Source: three-view drawing plus pictorial views. Frame: mm from the lowest corner of the part. A direction names the side the tool comes from. Give positions to 0.01 mm unless a question says otherwise; leave off trailing zeros. Order: outer loops, then holes, each group sorted by start corner. A loop starts at its lowest first (then second) coordinate and runs counter-clockwise, first axis right, second up.
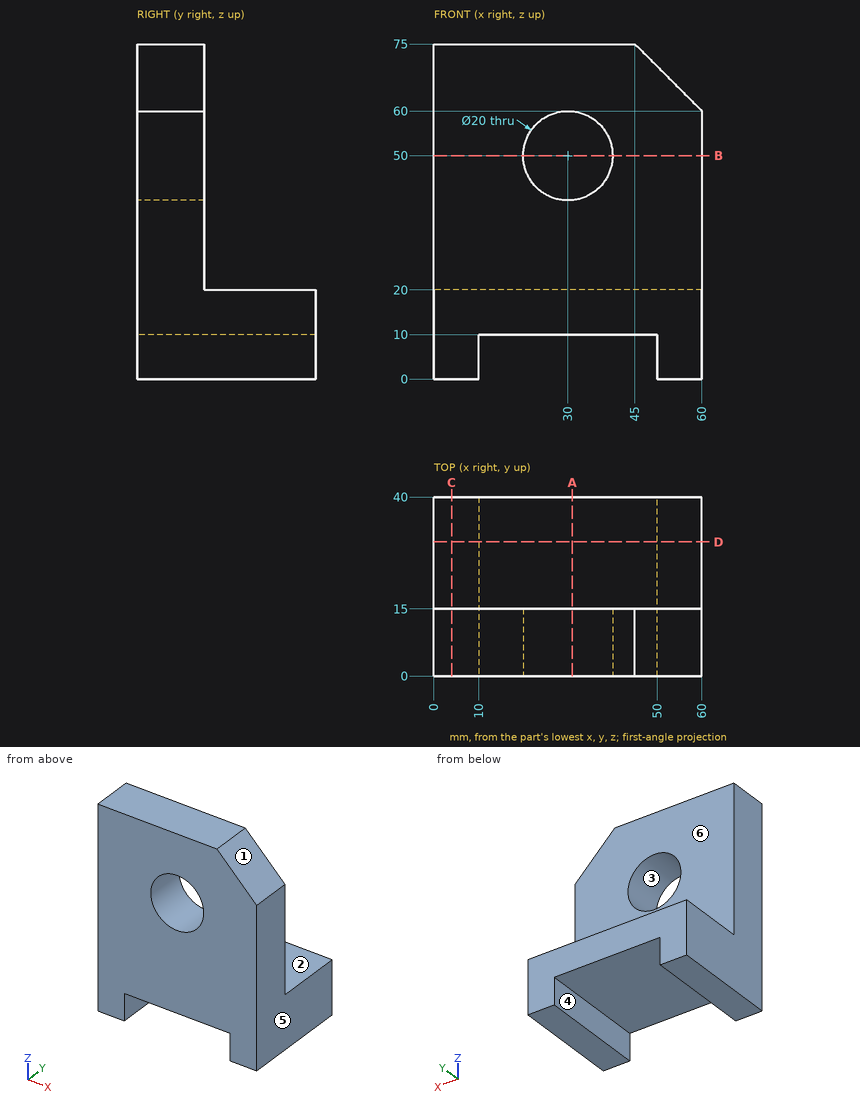
1) First-contact query: pin 1 Ø2 at (x, y) = (30.5, 31) entering from +Z; pin 2 Ø12 at (x, y) = (47, 33) entering from -Z; pin 3 Ø12 at (x, y) = (38.5, 27) entering from -Z; pin 4 Ø1.5 at (x, z) = (47.5, 34) entering from +Y. Flat tips, straight axial feed; report the tip coordinate or a pass-through.
Checks:
pin 1: stops at z = 20
pin 2: stops at z = 0
pin 3: stops at z = 10
pin 4: stops at y = 15
2) Reachability of the marked faces 4, 5 and 6 from +Z, -Z, +X, -X, +Y, -Y: full face, straight path, thin tool, end or side. Return the list, or none.
Checks:
face 4: -Z, +Y, -Y
face 5: +Z, -Z, +X, +Y, -Y
face 6: +Z, +X, -X, +Y
3) Section query C-C on x = 4. Output: boundary loops of the cut face in (y, z).
Checks:
outline: (0, 0) - (40, 0) - (40, 20) - (15, 20) - (15, 75) - (0, 75) - close
4) Ray query, L1, parallel to X at y = 10, z = 50; L2, parallel to Y at x = 21.5, z = 44; L3, parallel to Z at x = 3, y = 16. Return the intervals inside material, ascending.
Checks:
L1: x = 0 to 20, 40 to 60
L2: y = 0 to 15
L3: z = 0 to 20
5) Section query B-B on z = 50. Output: boundary loops of the cut face in (x, y), and give its area (3 significant figures).
Checks:
outline: (0, 0) - (20, 0) - (20, 15) - (0, 15) - close; (40, 0) - (60, 0) - (60, 15) - (40, 15) - close
area: 600 mm2
6) Pull-direction query (X, two-part tool) for the marked faces 1, 2 and 3; classes: +X half, -X half, draft (parallel to the pull), parting line (faces both ways), or undercut.
Checks:
face 1: +X half
face 2: draft
face 3: undercut
7) Section query A-A on x = 31. Output: boundary loops of the cut face in (y, z).
Checks:
outline: (0, 10) - (40, 10) - (40, 20) - (15, 20) - (15, 40.05) - (0, 40.05) - close; (0, 59.95) - (15, 59.95) - (15, 75) - (0, 75) - close
8) Section query D-D on y = 30. Output: boundary loops of the cut face in (x, z), and give its area (3 significant figures).
Checks:
outline: (0, 0) - (10, 0) - (10, 10) - (50, 10) - (50, 0) - (60, 0) - (60, 20) - (0, 20) - close
area: 800 mm2
